Check sheet for the modelled part. Datum: model origin and axes. Units: mm. Round coordinates to 2 decimals unless told otherwise and drop trailing zeros. Order: outer loops, then holes, each group sorted by start corner. A loop starts at its lowest first (then second) coordinate and runs counter-clockwise, first axis right, second up.
(1) Sectioned sample at A-A, the plane x = 93. Enter the section's corners in (y, z).
(2) Mould release check, pull along X, two halves, no side actions. Record for faces 1 (the cylindrical face through (85.847, -97.985, 7.888)), 2 (the flat face through (-2, 125, 8)), 3 (the flat face through (-125, -2, 8)), 4 (the flat face through (125, -2, 8)): released by +X, released by -X, zero draft, split by the parting line, or undercut.
(3) Sectioned sample at B-B, the plane z = 3. Enter the section's corners in (x, y).
(4) Sectioned sample at C-C, the plane y = 90. Enter the section's corners in (x, z), and give its area (3 significant figures).
(5) Thickness scan on probe 1 along Y at (x, z) = (90, 6.25); probe 2 along X at (y, z) = (-98, 8.75); probe 3 along Y at (x, z) = (85.5, 12.75). Record the ranges inside material, lowest first.
(6) Depth check by flat-ended pin: pin 1 (11 mm diameter, centred on x = 90, y = -90, fed in from -Z). Enter the tip coordinate at first touch or a pass-through.
```python
from build123d import *

# Parameters (mm, degrees)
F0_W     = 250
F0_H     = 250
F1_DEPTH = 16
F3_D     = 18
F3_DEPTH = 20


with BuildPart() as f1:
    # F0 (on Top) → F1 (new body)
    with BuildSketch(Plane.XY):
        Rectangle(F0_W, F0_H)
    extrude(amount=F1_DEPTH)

    # F3
    with Locations(Plane.XY.offset(16)):
        with Locations((-90, 90), (90, 90), (90, -90), (-90, -90)):
            Hole(F3_D / 2, depth=F3_DEPTH)


solid = f1.part
```
Derived:
1. outline: (-125, 0) - (-98.49, 0) - (-98.49, 16) - (-125, 16) - close; (-81.51, 0) - (81.51, 0) - (81.51, 16) - (-81.51, 16) - close; (98.49, 0) - (125, 0) - (125, 16) - (98.49, 16) - close
2. face 1: undercut
2. face 2: zero draft
2. face 3: released by -X
2. face 4: released by +X
3. outline: (-125, -125) - (125, -125) - (125, 125) - (-125, 125) - close; hole circle Ø18 at (-90, -90); hole circle Ø18 at (-90, 90); hole circle Ø18 at (90, -90); hole circle Ø18 at (90, 90)
4. outline: (-125, 0) - (-99, 0) - (-99, 16) - (-125, 16) - close; (-81, 0) - (81, 0) - (81, 16) - (-81, 16) - close; (99, 0) - (125, 0) - (125, 16) - (99, 16) - close
4. area: 3,420 mm2
5. probe 1: y = -125 to -99, -81 to 81, 99 to 125
5. probe 2: x = -125 to -94.12, -85.88 to 85.88, 94.12 to 125
5. probe 3: y = -125 to -97.79, -82.21 to 82.21, 97.79 to 125
6. pin 1: passes through
